from build123d import *

# Parameters (mm, degrees)
SKETCH010_W     = 47
SKETCH010_H     = 19.5
PAD006_DEPTH    = 1.5
SKETCH011_W     = 9
SKETCH011_H     = 7.7
PAD008_DEPTH    = 4
SKETCH012_R     = 1.2
POCKET003_DEPTH = 1.501
SKETCH013_W     = 2
SKETCH013_H     = 15.5
SKETCH013_H_2   = 7
PAD007_DEPTH    = 2
SKETCH004_W     = 2
SKETCH004_H     = 7
PAD005_DEPTH    = 8


with BuildPart() as part:
    # Sketch010 → Pad006 (new body)
    with BuildSketch(Plane.XY):
        with Locations((23.5, 9.75)):
            Rectangle(SKETCH010_W, SKETCH010_H)
    extrude(amount=PAD006_DEPTH)

    # Sketch011 (on Face6 of Pad006) → Pad008 (join)
    with BuildSketch(Plane.XY.offset(1.5)):
        with Locations((3, 9.75)):
            Rectangle(SKETCH011_W, SKETCH011_H)
    extrude(amount=PAD008_DEPTH)

    # Sketch012 (on Face5 of Pad008) → Pocket003 (cut, through all)
    with BuildSketch(Plane.XY.offset(1.5)):
        with Locations((11, 16.75)):
            Circle(SKETCH012_R)
        with Locations((11, 2.75)):
            Circle(SKETCH012_R)
    extrude(amount=-POCKET003_DEPTH, mode=Mode.SUBTRACT)

    # Sketch013 (on Face4 of Pocket003) → Pad007 (join)
    with BuildSketch(Plane(origin=(0, 0, 0), x_dir=(1, 0, 0), z_dir=(0, 0, -1))):
        with Locations((44, -9.75)):
            Rectangle(SKETCH013_W, SKETCH013_H)
        with Locations((16, -5.5)):
            Rectangle(SKETCH013_W, SKETCH013_H_2)
    extrude(amount=PAD007_DEPTH)

    # Sketch004 (on Face5 of Pad007) → Pad005 (join)
    with BuildSketch(Plane.XY.offset(1.5)):
        with Locations((16, 5.5)):
            Rectangle(SKETCH004_W, SKETCH004_H)
    extrude(amount=PAD005_DEPTH)


with BuildPart() as part_1:
    # Body001 placement: moved
    add(part.part.moved(Location((-69.5, -9.75, 4))))


solid = part_1.part
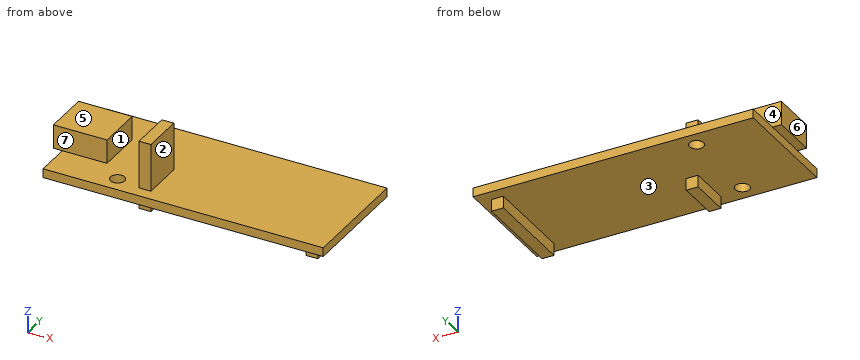
Could you check a few things on this model? Use its own coordinates, in mm. Face numbers are marked on the shaded views. A direction names the side the tool comes from. Give positions to 0.01 mm unless a question says otherwise; leave off trailing zeros. Order: outer loops, then holes, each group sorted by start corner. A loop starts at its lowest first (then second) coordinate and runs counter-clockwise, first axis right, second up. Notation, with made-up numbers: (-37.5, -26.75) -> (-26.5, -26.75) arc R16 cw to (-26.5, -2.75) -> close; hole circle Ø11 at (68, 54.5). An arc over 180 degrees is marked (long way). Answer in a Markdown table with one row per item. Add a question column.
Item 1: We'd pull the mould along X, two halves only. Please class the marked faces 1, 2, 3 and 4: pulls with the +X half, pulls with the -X half, needs draft (parallel to the pull), parting line crosses it, or undercut.
Item 2: Imagine slicing it at C-C (x = -58.5). List the corners of the cut face in (y, z) for me.
Item 3: Imagine slicing it at A-A (y = 7). List the corners of the cut face in (x, z) for me, and give its area (3 significant figures).
Item 4: For the marked faces 5, 6 and 7, which set-ups out of +Z, -Z, +X, -X, +Y, -Y let a thin tool reach every point of the face, with its end or its side?
Item 5: Imagine slicing it at D-D (y = -2.5). List the corners of the cut face in (x, z) for me.
Item 6: Imagine slicing it at B-B (z = 6.75). List the corners of the cut face in (x, y) for me, and give its area (3 significant figures).
Item 7: I'm going to push flat-ended pins straight in: P1, Ø4.5, axis at x = -67, z = 8.5, coming from the +Y side; P2, Ø1.6, axis at y = -3, z = 3.5, coming from the +X side; P3, Ø0.6, axis at x = -53.5, z = 3, coming from the -Y side; P4, Ø6, axis at x = -46, y = 4, coming from the -Z side. Where does each tip first touch, or does it pass through?
Item 8: Please list where these lines run through material, in increasing order: probe 1 along Y at (x, z) = (-58.5, 5.25); probe 2 along X at (y, z) = (-1.25, 9.75); probe 3 along Z at (x, y) = (-39, -5).
Result:
| question | item | result |
|---|---|---|
| 1 | face 1 | undercut |
| 1 | face 2 | pulls with the +X half |
| 1 | face 3 | undercut |
| 1 | face 4 | needs draft |
| 2 | outline | (-9.75, 4) -> (-8.2, 4) -> (-8.2, 5.5) -> (-9.75, 5.5) -> close; (-5.8, 4) -> (5.8, 4) -> (5.8, 5.5) -> (-5.8, 5.5) -> close; (8.2, 4) -> (9.75, 4) -> (9.75, 5.5) -> (8.2, 5.5) -> close |
| 3 | outline | (-69.5, 4) -> (-59.7, 4) -> (-59.7, 5.5) -> (-69.5, 5.5) -> close; (-57.3, 4) -> (-26.5, 4) -> (-26.5, 2) -> (-24.5, 2) -> (-24.5, 4) -> (-22.5, 4) -> (-22.5, 5.5) -> (-57.3, 5.5) -> close |
| 3 | area | 70.9 mm2 |
| 4 | face 5 | +Z, -X, +Y, -Y |
| 4 | face 6 | +Z, -Z, -X, +Y, -Y |
| 4 | face 7 | +Z, -X, -Y |
| 5 | outline | (-71, 5.5) -> (-69.5, 5.5) -> (-69.5, 4) -> (-54.5, 4) -> (-54.5, 2) -> (-52.5, 2) -> (-52.5, 4) -> (-26.5, 4) -> (-26.5, 2) -> (-24.5, 2) -> (-24.5, 4) -> (-22.5, 4) -> (-22.5, 5.5) -> (-52.5, 5.5) -> (-52.5, 13.5) -> (-54.5, 13.5) -> (-54.5, 5.5) -> (-62, 5.5) -> (-62, 9.5) -> (-71, 9.5) -> close |
| 6 | outline | (-71, -3.85) -> (-62, -3.85) -> (-62, 3.85) -> (-71, 3.85) -> close; (-54.5, -7.75) -> (-52.5, -7.75) -> (-52.5, -0.75) -> (-54.5, -0.75) -> close |
| 6 | area | 83.3 mm2 |
| 7 | P1 | y = 3.85 |
| 7 | P2 | x = -22.5 |
| 7 | P3 | y = -7.75 |
| 7 | P4 | z = 4 |
| 8 | probe 1 | -9.75 to -8.2, -5.8 to 5.8, 8.2 to 9.75 |
| 8 | probe 2 | -54.5 to -52.5 |
| 8 | probe 3 | 4 to 5.5 |
